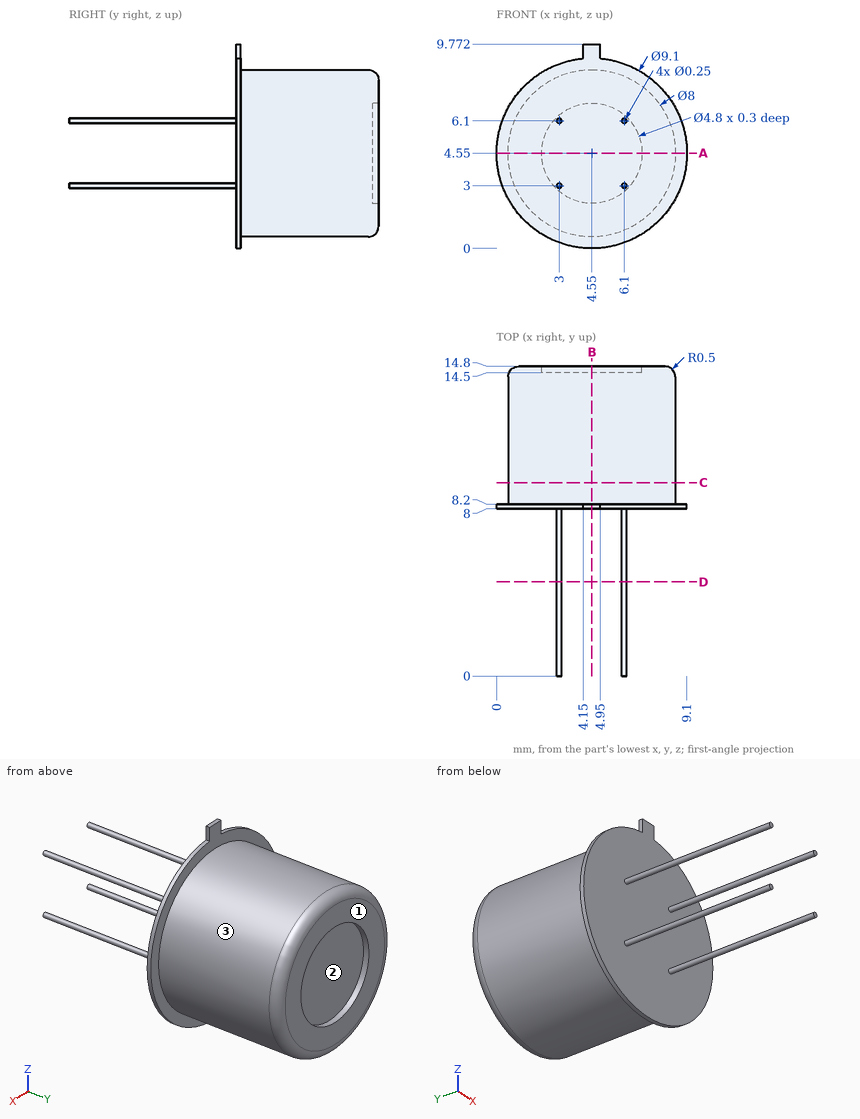
Answer from the drawing. Dimensions are ordinates in mm from the lowest x, y and z of the part. Coordinates: 2 decimals unless noted, no trailing zeros. Write each loop counter-clockwise with the first axis right and the second up, starting at its lowest first coordinate (ties: lowest second). Pieces come first, ordered by that corner, then holes. Notation, with made-up numbers: (35.25, 55.25) - (61.25, 55.25) arc R14 ccw to (61.25, 64.25) - close; hole circle Ø9 at (3, 16). An arc over 180 degrees is marked (long way). Return JSON: item names as keys, results as strings.
1. For a pull along X with two mould halves and no side action, classify the marked faces 1, 2 and 3 as +X half, -X half, draft (parallel to the pull), parting line (faces both ways), or undercut.
Final values:
{"face 1": "draft", "face 2": "undercut", "face 3": "parting line"}
2. The part is cut by section D-D on y = 4.5. Count the separate pieces of the cut face and the enclosed holes in it.
Final values:
{"separate pieces": "4", "enclosed holes": "0"}
3. The part is cut by section B-B on x = 4.55. Determine the outline of the cut face in (y, z).
Final values:
{"outline": "(8, 0) - (8.2, 0) - (8.2, 0.55) - (14.3, 0.55) arc R0.5 ccw to (14.8, 1.05) - (14.8, 2.15) - (14.5, 2.15) - (14.5, 6.95) - (14.8, 6.95) - (14.8, 8.05) arc R0.5 ccw to (14.3, 8.55) - (8.2, 8.55) - (8.2, 9.77) - (8, 9.77) - close"}
4. Consider line 1 along Y through (x, z) = (1.75, 4.5); line 2 along Y through (x, z) = (1, 6.5); line 3 along X through (y, z) = (14.6, 4.55). Determine where each line is inside the solid, lowest interval first.
Final values:
{"line 1": "8 to 14.8", "line 2": "8 to 8.2", "line 3": "0.65 to 2.15, 6.95 to 8.45"}
5. Each of these flat-tipped pins is pushed along its axis until it touches: pin 1 Ø4 at (x, y) = (8, 8.5) entering from -Z (1 decimal); pin 2 Ø1.4 at (x, z) = (4.5, 3.5) entering from +Y; pin 3 Ø4 at (y, z) = (13, 4) entering from +X. Where does it stop, or does it pass through?
Final values:
{"pin 1": "z = 0.2", "pin 2": "y = 14.5", "pin 3": "x = 8.55"}
6. The part is cut by section C-C on y = 9.25. Determine the outline of the cut face in (x, z), then the cut area to 3 significant figures.
Final values:
{"outline": "circle Ø8 at (4.55, 4.55)", "area": "50.3 mm^2"}
7. The part is cut by section A-A on z = 4.55. Determine the outline of the cut face in (x, y).
Final values:
{"outline": "(0, 8) - (9.1, 8) - (9.1, 8.2) - (8.55, 8.2) - (8.55, 14.3) arc R0.5 ccw to (8.05, 14.8) - (6.95, 14.8) - (6.95, 14.5) - (2.15, 14.5) - (2.15, 14.8) - (1.05, 14.8) arc R0.5 ccw to (0.55, 14.3) - (0.55, 8.2) - (0, 8.2) - close"}
